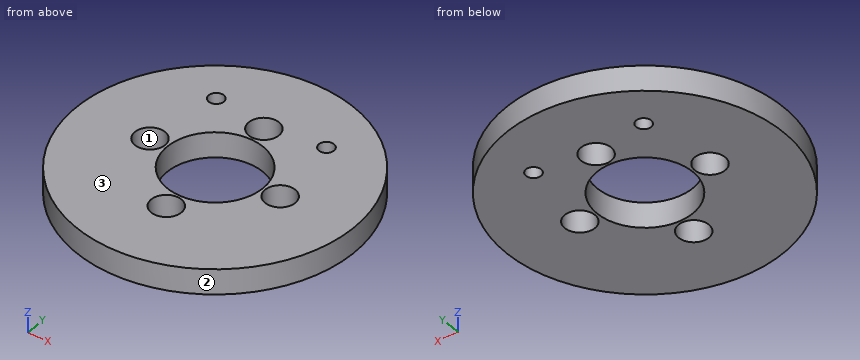
from build123d import *

# Parameters (mm, degrees)
ESQUISSE1_R             = 27.5
ESQUISSE1_R_2           = 9.5
BOSS_EXTRU_1_DEPTH      = 5
ESQUISSE2_R             = 3
ESQUISSE2_R_2           = 1.5
ENL_V_MAT_EXTRU_1_DEPTH = 5


with BuildPart() as part:
    # Esquisse1 → Boss.-Extru.1 (new body)
    with BuildSketch(Plane.XY):
        Circle(ESQUISSE1_R)
        Circle(ESQUISSE1_R_2, mode=Mode.SUBTRACT)
    extrude(amount=BOSS_EXTRU_1_DEPTH)

    # Esquisse2 → Enlèv. mat.-Extru.1 (cut)
    with BuildSketch(Plane.XY.offset(5)):
        with Locations((-13, 0)):
            Circle(ESQUISSE2_R)
        with Locations((0, 13)):
            Circle(ESQUISSE2_R)
        with Locations((13, 0)):
            Circle(ESQUISSE2_R)
        with Locations((0, -13)):
            Circle(ESQUISSE2_R)
        with Locations((11, 15)):
            Circle(ESQUISSE2_R_2)
        with Locations(Location((-11, 15, 0), (0, 0, 180))):
            Circle(ESQUISSE2_R_2)
    extrude(amount=-ENL_V_MAT_EXTRU_1_DEPTH, mode=Mode.SUBTRACT)


solid = part.part
Could you check a few things on this model? Use its own coordinates, in mm. Face numbers are marked on the shaded views. Coordinates: 2 decimals unless noted, no trailing zeros. Write each loop counter-clockwise with the first axis right and the second up, starting at its lowest first coordinate (ties: lowest second). Pieces come first, ordered by that corner, then holes. Notation, with made-up numbers: M 54,84 L 111,84 A23 ccw 111,92 Z; hole C 33.25,25.25 d9. An arc over 180 degrees is marked long. One line per question, with ' | ' between items.
1) Imagine slicing it at A-A, the plane x = 0. Write out the boundary of the cut face in (y, z).
Checks:
outline: M -27.5,0 L -16,0 L -16,5 L -27.5,5 Z; M -10,0 L -9.5,0 L -9.5,5 L -10,5 Z; M 9.5,0 L 10,0 L 10,5 L 9.5,5 Z; M 16,0 L 27.5,0 L 27.5,5 L 16,5 Z
2) Imagine slicing it at B-B, the plane y = 15. Write out the boundary of the cut face in (x, z).
Checks:
outline: M -23.05,0 L -12.5,0 L -12.5,5 L -23.05,5 Z; M -9.5,0 L -2.24,0 L -2.24,5 L -9.5,5 Z; M 2.24,0 L 9.5,0 L 9.5,5 L 2.24,5 Z; M 12.5,0 L 23.05,0 L 23.05,5 L 12.5,5 Z
3) For pin 1 Ø1.5 at (x, z) = (20, 1.5) entering from -Y; pin 2 Ø2.5 at (x, y) = (11, 15) entering from -Z; pin 3 Ø1 at (y, z) = (1.5, 4.5) entering from +X; pin 4 Ø1 at (x, z) = (-18.5, 2.5) entering from -Y, each with a flat end and sliding along its axis, tell me the tip position at first contact or that it passes through.
Checks:
pin 1: y = -19.64 | pin 2: through | pin 3: x = 27.48 | pin 4: y = -20.79
4) Imagine slicing it at D-D, the plane y = 6. Write out the boundary of the cut face in (x, z).
Checks:
outline: M -26.84,0 L -7.37,0 L -7.37,5 L -26.84,5 Z; M 7.37,0 L 26.84,0 L 26.84,5 L 7.37,5 Z
5) Imagine slicing it at C-C, the plane z = 2.2. Write out the boundary of the cut face in (x, y).
Checks:
outline: C 0,0 d55; hole C -13,0 d6; hole C -11,15 d3; hole C 0,0 d19; hole C 0,-13 d6; hole C 0,13 d6; hole C 11,15 d3; hole C 13,0 d6
6) I need wall thicknesses on probe 1 along Y at (x, z) = (0, 1.7); probe 2 along Y at (x, z) = (1, 4.15); probe 3 along Y at (x, z) = (11, 3.15). Which ranges of each line are inside material? Lowest first, please. Write a range as [from, to].
Checks:
probe 1: [-27.5, -16], [-10, -9.5], [9.5, 10], [16, 27.5] | probe 2: [-27.48, -15.83], [-10.17, -9.45], [9.45, 10.17], [15.83, 27.48] | probe 3: [-25.2, -2.24], [2.24, 13.5], [16.5, 25.2]
7) If we mould it in two halves opening along Y, with no side actions, what happens to the marked faces 1, 2 and 3? For each: released by +Y, released by -Y, zero draft, split by the parting line, or undercut.
Checks:
face 1: undercut | face 2: split by the parting line | face 3: zero draft
